```python
from build123d import *

# Parameters (mm, degrees)
BASE_FLANGE1_DEPTH = 300
CUT_EXTRUDE1_DEPTH = 10
LPATTERN1_COUNT    = 11
LPATTERN1_PITCH    = 25


# Sheet-metal steps are written as plain solids
with BuildPart() as part:
    # Sketch1 → Base-Flange1 (new body)
    with BuildSketch(Plane.XY):
        with BuildLine():
            Line((0, 0), (3.2634, 0))
            ThreePointArc((3.2634, 0), (4.491361636, -0.508638364), (5, -1.7366))
            Line((5, -1.7366), (5, -6.7634))
            ThreePointArc((5, -6.7634), (5.215745145, -7.284254855), (5.7366, -7.5))
            Line((5.7366, -7.5), (31.2634, -7.5))
            ThreePointArc((31.2634, -7.5), (31.784254855, -7.284254855), (32, -6.7634))
            Line((32, -6.7634), (32, -1.7366))
            ThreePointArc((32, -1.7366), (32.508638364, -0.508638364), (33.7366, 0))
            Line((33.7366, 0), (37, 0))
            Line((37, 0), (37, -1))
            Line((37, -1), (33.7366, -1))
            ThreePointArc((33.7366, -1), (33.215745145, -1.215745145), (33, -1.7366))
            Line((33, -1.7366), (33, -6.7634))
            ThreePointArc((33, -6.7634), (32.491361636, -7.991361636), (31.2634, -8.5))
            Line((31.2634, -8.5), (5.7366, -8.5))
            ThreePointArc((5.7366, -8.5), (4.508638364, -7.991361636), (4, -6.7634))
            Line((4, -6.7634), (4, -1.7366))
            ThreePointArc((4, -1.7366), (3.784254855, -1.215745145), (3.2634, -1))
            Line((3.2634, -1), (0, -1))
            Line((0, -1), (0, 0))
        make_face()
    extrude(amount=BASE_FLANGE1_DEPTH)

    # Sketch6 → Cut-Extrude1 (cut)
    with BuildSketch(Plane(origin=(0, -7.5, 0), x_dir=(1, 0, 0), z_dir=(0, 1, 0))):
        with BuildLine():
            Line((21.3866, -273), (21.3866, -287))
            ThreePointArc((21.3866, -287), (18.2366, -290.15), (15.0866, -287))
            Line((15.0866, -287), (15.0866, -273))
            ThreePointArc((15.0866, -273), (18.2366, -269.85), (21.3866, -273))
        make_face()
    cut_extrude1 = extrude(amount=-CUT_EXTRUDE1_DEPTH, mode=Mode.SUBTRACT)

    # LPattern1: Cut-Extrude1 ×11
    with Locations(*[(0, 0, -i * LPATTERN1_PITCH) for i in range(1, LPATTERN1_COUNT)]):
        add(cut_extrude1, mode=Mode.SUBTRACT)


solid = part.part
```
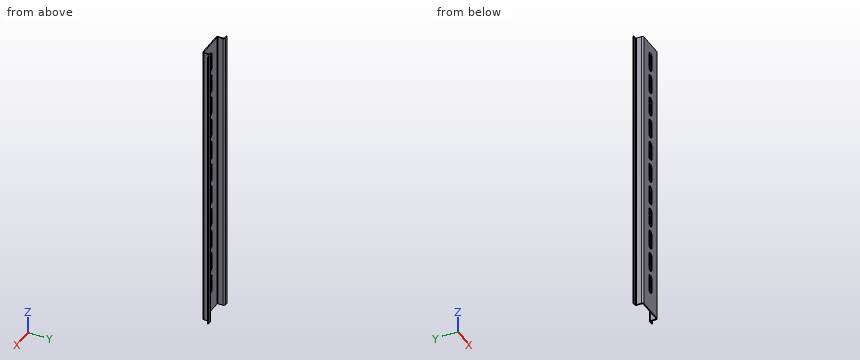
Work out the finished part from the listing and answer in its coordinate system (mm). Round coordinates to 2 decimals unless told otherwise and drop trailing zeros. Write each loop counter-clockwise with the first axis right and the second up, starting at its lowest first coordinate (ties: lowest second). Pieces come first, ordered by that corner, then holes.
1) A cutting plane is placed at B-B on y = -4.75. Determine the outline of the cut face in (x, z), and give its area (3 significant figures).
2) Consider probe 1 along X at (y, z) = (-4, 177); probe 2 along Y at (x, z) = (23, 267.5); probe 3 along X at (y, z) = (-1.25, 104.5). Determine where each line is inside the solid, lowest interval first.
3) Flat-ended cylindrical pins translate along their axes: P1, Ø0.8, axis at y = -8, z = 31, coming from the +X side; P2, Ø4, axis at x = 12.5, z = 248, coming from the +Y side; P3, Ø1.5, axis at y = -3, z = 135, coming from the -X side. Find the tip coordinate at first contact, or state that the pin passes through.
4) A cutting plane is placed at A-A on z = 56. Determine the outline of the cut face in (x, y), and give its area (3 significant figures).
5) A cutting plane is placed at C-C on x = 18. Give the number of separate pieces and of enclosed holes in the cut face, and give its area (3 significant figures).
Entries:
1. outline: (4, 0) - (5, 0) - (5, 300) - (4, 300) - close; (32, 0) - (33, 0) - (33, 300) - (32, 300) - close
1. area: 600 mm2
2. probe 1: x = 4 to 5, 32 to 33
2. probe 2: y = -8.5 to -7.5
2. probe 3: x = 3.82 to 4.93, 32.07 to 33.18
3. P1: stops at x = 32.79
3. P2: stops at y = -7.5
3. P3: stops at x = 4
4. outline: (0, -1) - (3.26, -1) arc R0.74 cw to (4, -1.74) - (4, -6.76) arc R1.74 ccw to (5.74, -8.5) - (15.09, -8.5) - (15.09, -7.5) - (5.74, -7.5) arc R0.74 cw to (5, -6.76) - (5, -1.74) arc R1.74 ccw to (3.26, 0) - (0, 0) - close; (21.39, -8.5) - (31.26, -8.5) arc R1.74 ccw to (33, -6.76) - (33, -1.74) arc R0.74 cw to (33.74, -1) - (37, -1) - (37, 0) - (33.74, 0) arc R1.74 ccw to (32, -1.74) - (32, -6.76) arc R0.74 cw to (31.26, -7.5) - (21.39, -7.5) - close
4. area: 43.6 mm2
5. separate pieces: 12
5. enclosed holes: 0
5. area: 76.9 mm2
